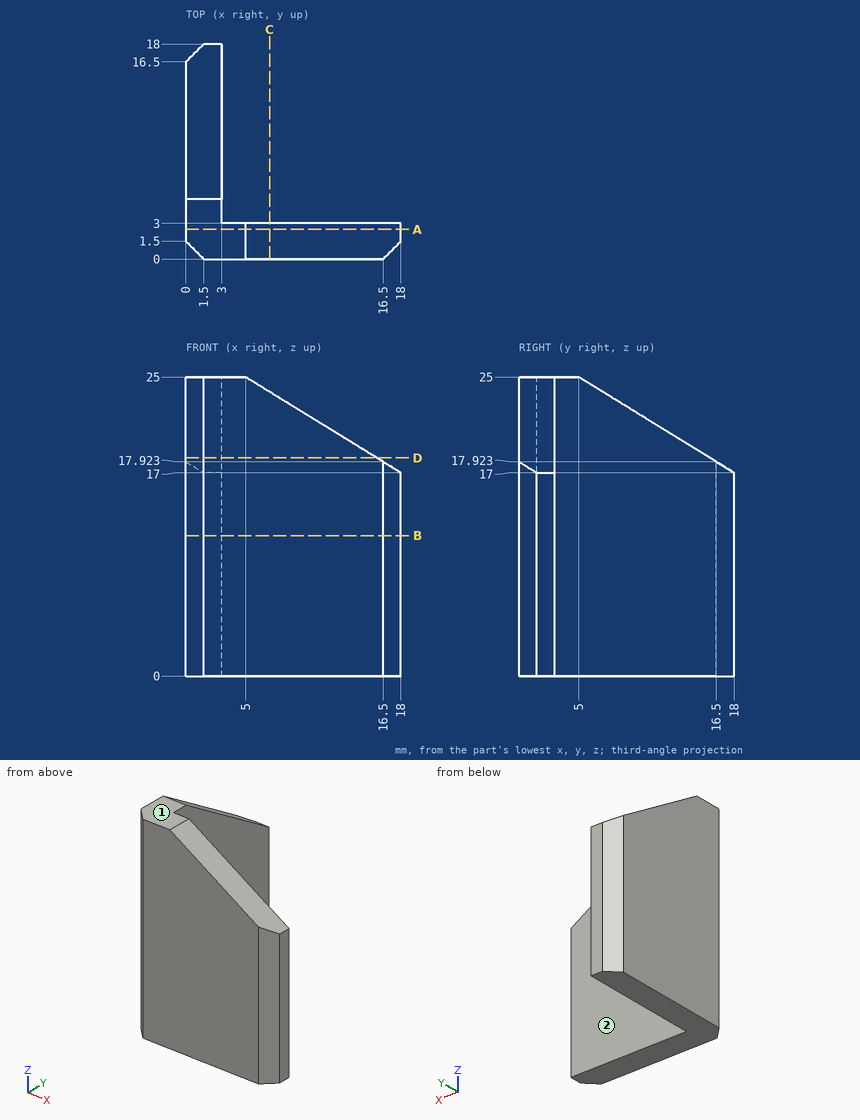
Verification items for this drawing (mm, ordinates from the low corner). A direction names the side the tool comes from. Coordinates: 2 decimals unless noted, no trailing zeros. Write each loop counter-clockwise with the first axis right and the second up, starting at its lowest first coordinate (ties: lowest second). Pieces come first, ordered by that corner, then holes. Notation, with made-up numbers: M 86.5,55 L 123.5,55 A22 ccw 123.5,93 Z; hole C -23.75,41.5 d3. An arc over 180 degrees is marked long. Use one line per item in the form item = value. Start each with the question number.
1) Section check B-B on z = 11.75. Enter the section's corners in (x, y).
2) Section check A-A on y = 2.5. Enter the section's corners in (x, z).
3) Section check D-D on z = 18.25. Enter the section's corners in (x, y), and give its area (3 significant figures).
4) Set-up check for the marked faces 1 and 2: record each of +Z, -Z, +X, -X, +Y, -Y from which the full face is reachable in a straight line by a thin tool's end or side.
5) Thickness scan on probe 1 along X at (y, z) = (9, 6.75); probe 2 along Y at (x, z) = (2, 19). Record the ranges inside material, lowest first. Write a range as from..to.
6) Go/stop test with flat-tipped pins: pin 1 Ø8 at (x, z) = (3, 22) entering from +Y (3 decimals); pin 2 Ø4 at (y, z) = (8, 21) entering from +X; pin 3 Ø7.5 at (x, z) = (8, 7) entering from +Y. Record where each tip stops, or that it passes through.
7) Section check C-C on x = 7. Enter the section's corners in (y, z), and give its area (3 significant figures).
Responses:
q1.outline = M 0,1.5 L 1.5,0 L 16.5,0 L 18,1.5 L 18,3 L 3,3 L 3,18 L 1.5,18 L 0,16.5 Z
q2.outline = M 0,0 L 18,0 L 18,17 L 5,25 L 0,25 Z
q3.outline = M 0,1.5 L 1.5,0 L 15.97,0 L 15.97,3 L 3,3 L 3,15.97 L 0,15.97 Z
q3.area = 85.7 mm2
q4.face_1 = +Z, +X, -X, +Y, -Y
q4.face_2 = +Z, -Z, +X, +Y
q5.probe_1 = 0..3
q5.probe_2 = 0..14.75
q6.pin_1 = 16.375
q6.pin_2 = 3
q6.pin_3 = 3
q7.outline = M 0,0 L 3,0 L 3,23.77 L 0,23.77 Z
q7.area = 71.3 mm2
